The drawing under review shows one solid part. Ordinate dimensions are in mm from its lowest x, y, z. A direction names the side the tool comes from. Give positions to 0.01 mm unless a question says otherwise; leave off trailing zeros. Loops run counter-clockwise (first coordinate to the right, second up) from the corner with the lowest first, then second, coordinate; pieces in that order, holes last. Notation, with made-up numbers: (20.5, 19) -> (53.5, 19) arc R24 ccw to (53.5, 36) -> close; hole circle Ø4 at (23, 89.5). An arc over 180 degrees is marked (long way). Answer in a Markdown table with one row per item. Add a question column.
(1) For line 1 (X direction, y = 56.5, z = 33); line 2 (X direction, y = 52.5, z = 9.5); line 3 (Z direction, x = 378, y = 7.5), list the stretches that pass through material, from the lowest coordinate up.
(2) Consider section B-B on y = 11. Write out the cut boundary in (x, z).
(3) For the marked faces 1 and 2, list the 3-axis set-ups (+Z, -Z, +X, -X, +Y, -Y) from which the entire face can be reached by the end or side of a thin tool; tool diameter is ignored.
(4) Consider section A-A on z = 32. Write out the cut boundary in (x, y).
(5) Consider section C-C on x = 387. Write out the cut boundary in (y, z), then the cut area to 3 significant figures.
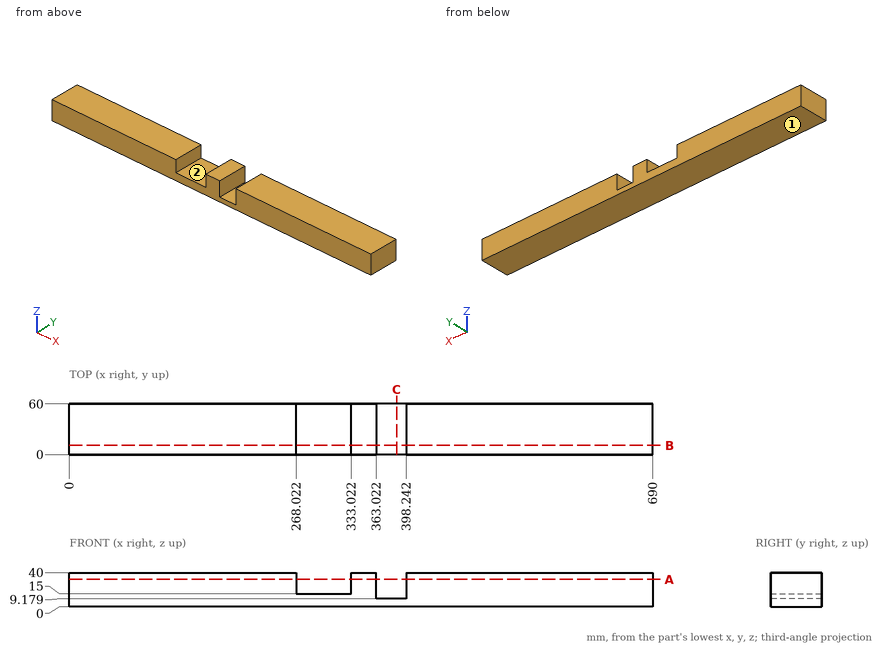
Values follow:
| question | item | result |
|---|---|---|
| 1 | line 1 | 0 to 268.02, 333.02 to 363.02, 398.24 to 690 |
| 1 | line 2 | 0 to 363.02, 398.24 to 690 |
| 1 | line 3 | 0 to 9.18 |
| 2 | outline | (0, 0) -> (690, 0) -> (690, 40) -> (398.24, 40) -> (398.24, 9.18) -> (363.02, 9.18) -> (363.02, 40) -> (333.02, 40) -> (333.02, 15) -> (268.02, 15) -> (268.02, 40) -> (0, 40) -> close |
| 3 | face 1 | -Z, +X, -X, +Y, -Y |
| 3 | face 2 | +Z, +Y, -Y |
| 4 | outline | (0, 0) -> (268.02, 0) -> (268.02, 60) -> (0, 60) -> close; (333.02, 0) -> (363.02, 0) -> (363.02, 60) -> (333.02, 60) -> close; (398.24, 0) -> (690, 0) -> (690, 60) -> (398.24, 60) -> close |
| 5 | outline | (0, 0) -> (60, 0) -> (60, 9.18) -> (0, 9.18) -> close |
| 5 | area | 551 mm2 |
